from build123d import *

# Parameters (mm, degrees)
SKETCH_2_R      = 8.5
SKETCH_2_R_2    = 2.6
SKETCH_2_R_3    = 1
EXTRUDE_1_DEPTH = 2
SKETCH_3_R      = 3.5
SKETCH_3_R_2    = 2.6
EXTRUDE_2_DEPTH = 2
SKETCH_4_R      = 3.5
SKETCH_4_R_2    = 2.6
EXTRUDE_3_DEPTH = 5
CHAMFER_1_SIZE  = 0.5


with BuildPart() as part:
    # Эскиз2 → Бобышка-Вытянуть1 (new body)
    with BuildSketch(Plane.XY):
        Circle(SKETCH_2_R)
        Circle(SKETCH_2_R_2, mode=Mode.SUBTRACT)
        with Locations((-6, 0)):
            Circle(SKETCH_2_R_3, mode=Mode.SUBTRACT)
        with Locations((0, 6)):
            Circle(SKETCH_2_R_3, mode=Mode.SUBTRACT)
        with Locations((6, 0)):
            Circle(SKETCH_2_R_3, mode=Mode.SUBTRACT)
        with Locations((0, -6)):
            Circle(SKETCH_2_R_3, mode=Mode.SUBTRACT)
    extrude(amount=EXTRUDE_1_DEPTH)

    # Эскиз3 → Бобышка-Вытянуть2 (add)
    with BuildSketch(Plane.XY.offset(2)):
        Circle(SKETCH_3_R)
        Circle(SKETCH_3_R_2, mode=Mode.SUBTRACT)
    extrude(amount=EXTRUDE_2_DEPTH)

    # Эскиз4 → Бобышка-Вытянуть3 (add)
    with BuildSketch(Plane(origin=(0, 0, 0), x_dir=(-1, 0, 0), z_dir=(0, 0, -1))):
        Circle(SKETCH_4_R)
        Circle(SKETCH_4_R_2, mode=Mode.SUBTRACT)
    extrude(amount=EXTRUDE_3_DEPTH)

    # Фаска1
    chamfer_1_edges = [part.edges().sort_by_distance(p)[0] for p in [
        (3.5, 0, -5),
    ]]
    chamfer(chamfer_1_edges, length=CHAMFER_1_SIZE)


solid = part.part
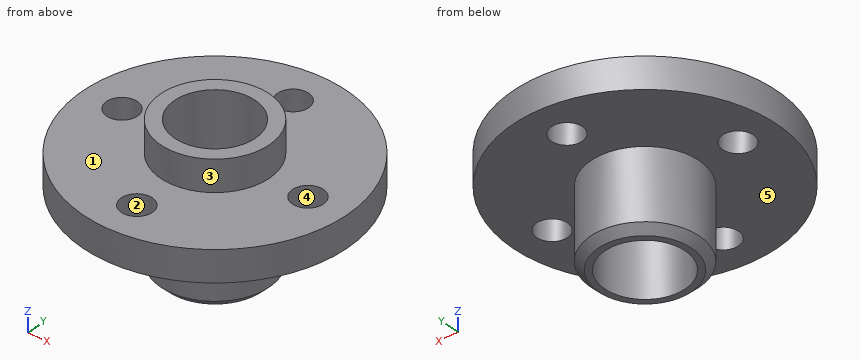
Verification items for the finished model (mm, model axes). Face numbers are marked on the shaded views. A direction names the side the tool comes from. Coordinates: 2 decimals unless noted, no trailing zeros. Order: outer loops, then holes, each group sorted by start corner. A loop starts at its lowest first (then second) coordinate and runs counter-clockwise, first axis right, second up. Notation, with made-up numbers: M -28,-28.75 L -1,-28.75 A25 ccw -1,9.25 Z; hole C 83,-12.75 d7. An arc over 180 degrees is marked long. One line per item, written item: value. Start each with the question number.
Item 1: Depth check by flat-ended pin: P1, Ø4, axis at y = 3, z = -3.5, coming from the +X side; P2, Ø2.5, axis at x = 6, y = 0, coming from the +Z side; P3, Ø2.5, axis at x = 0, y = 6, coming from the -Z side; P4, Ø8, axis at x = -5, y = -5, coming from the +Z side. Enter the tip coordinate at first touch or a pass-through.
Item 2: Thickness scan on probe 1 along Y at (x, z) = (0, 0.85); probe 2 along Y at (x, z) = (0, -2.3); probe 3 along Z at (x, y) = (-0.25, 4.75). Record the ranges inside material, lowest first.
Item 3: Sectioned sample at D-D on z = 2.25. Record the cut outline in (x, y).
Item 4: Mould release check, pull along Y, two halves, no side actions. Record for the marked faces 1, 2 and 3: pulls with the +Y half, pulls with the -Y half, needs draft (parallel to the pull), parting line crosses it, or undercut.
Item 5: Sectioned sample at A-A on y = 0. Record the cut outline in (x, z).
Item 6: Sectioned sample at B-B on y = 6. Record the cut outline in (x, z).
Item 7: Access from +Z, -Z, +X, -X, +Y, -Y to the whole of each face (thin tool, end or side, straight path). Record for the marked faces 4 and 5.
Calculated:
1. P1: x = 3.35
1. P2: z = 2
1. P3: z = 0
1. P4: z = 4
2. probe 1: -8.5 to -7, -5 to -2.6, 2.6 to 5, 7 to 8.5
2. probe 2: -3.5 to -2.6, 2.6 to 3.5
2. probe 3: 0 to 2
3. outline: C 0,0 d7; hole C 0,0 d5.2
4. face 1: needs draft
4. face 2: undercut
4. face 3: parting line crosses it
5. outline: M -8.5,0 L -7,0 L -7,2 L -8.5,2 Z; M -5,0 L -3.5,0 L -3.5,-4.5 L -3,-5 L -2.6,-5 L -2.6,4 L -3.5,4 L -3.5,2 L -5,2 Z; M 2.6,-5 L 3,-5 L 3.5,-4.5 L 3.5,0 L 5,0 L 5,2 L 3.5,2 L 3.5,4 L 2.6,4 Z; M 7,0 L 8.5,0 L 8.5,2 L 7,2 Z
6. outline: M -6.02,0 L -1,0 L -1,2 L -6.02,2 Z; M 1,0 L 6.02,0 L 6.02,2 L 1,2 Z
7. face 4: +Z, -Z
7. face 5: -Z
